Build history of the part. All positions in model axes, mm. Face numbers are marked on the shaded views. A direction names the side the tool comes from. Give positions to 0.01 mm unless a question says otherwise; leave off trailing zeros. Write each loop counter-clockwise with the first axis right and the second up, starting at its lowest first coordinate (ties: lowest second). Pieces come first, ordered by that corner, then holes. Notation, with made-up numbers: (14, 24) -> (35, 24) arc R32 cw to (35, 60) -> close; hole circle Ø1 at (-7, 53). An arc over 180 degrees is marked (long way). One line per question, with ' | ' between items. Start each with the question number.
(1) Tool access for the marked faces 4, 5 and 6: list every direction of +Z, -Z, +X, -X, +Y, -Y with a clear straight run to the whole face (end or side of a thin tool).
(2) Pull direction Z, two halves, no side cores. Call the marked faces 1, 2 and 3: released by +Z, released by -Z, zero draft, split by the parting line, or undercut.
(3) Band-saw the part on A-A, the plane y = -2.25. Give the cut face in (x, z).
(4) Drill centre lines: probe 1 along X at (y, z) = (-2.45, 0); probe 2 along X at (y, z) = (-0.5, 5). Where is each one in solid material? Low to high. Write a range as from..to.
(5) Band-saw the part on B-B, the plane y = 2. Count the separate pieces of the cut face and the enclosed holes in it, and give its area (3 significant figures).
(6) Pin check, flat tips, straight feed: P1, Ø2, axis at x = -0.5, y = 9, coming from the -Z side; P2, Ø1.5, axis at y = 1, z = -6, coming from the -X side; P3, Ø10, axis at x = 13, z = -12, coming from the +Y side; P4, Ø21.5, axis at x = 0.5, z = 3, coming from the -Y side. Stop position of each tip, or through.
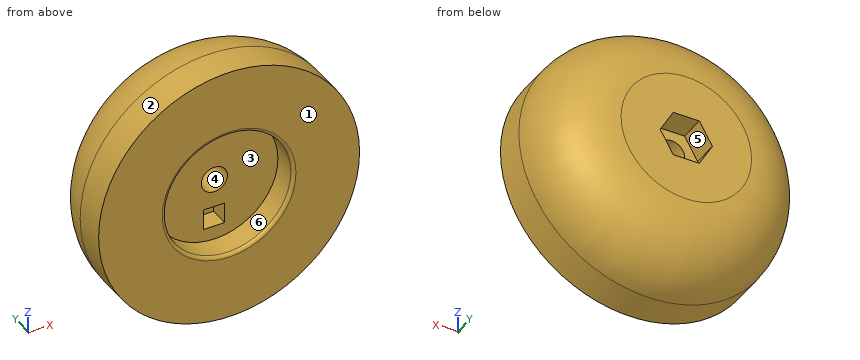
from build123d import *

# Parameters (mm, degrees)
SKETCH1_R           = 9.75
SKETCH1_R_2         = 2
BOSS_EXTRUDE1_DEPTH = 3
SKETCH2_W           = 3.2
SKETCH2_H           = 3.2
CUT_EXTRUDE1_DEPTH  = 3
SKETCH3_R           = 20
BOSS_EXTRUDE2_DEPTH = 8
SKETCH4_R           = 20
SKETCH4_R_2         = 9.75
BOSS_EXTRUDE3_DEPTH = 7
FILLET2_R           = 10
SKETCH5_R           = 2
CUT_EXTRUDE2_DEPTH  = 9
CUT_EXTRUDE3_DEPTH  = 4
FILLET3_R           = 0.5


with BuildPart() as part:
    # Sketch1 → Boss-Extrude1 (new body)
    with BuildSketch(Plane(origin=(0, 0, 0), x_dir=(1, 0, 0), z_dir=(0, 1, 0))):
        Circle(SKETCH1_R)
        Circle(SKETCH1_R_2, mode=Mode.SUBTRACT)
    extrude(amount=BOSS_EXTRUDE1_DEPTH)

    # Sketch2 → Cut-Extrude1 (cut)
    with BuildSketch(Plane.XZ):
        with Locations((-0.030329448, -6.016441714)):
            Rectangle(SKETCH2_W, SKETCH2_H)
    extrude(amount=-CUT_EXTRUDE1_DEPTH, mode=Mode.SUBTRACT)

    # Sketch3 → Boss-Extrude2 (add)
    with BuildSketch(Plane(origin=(0, 3, 0), x_dir=(1, 0, 0), z_dir=(0, 1, 0))):
        Circle(SKETCH3_R)
    extrude(amount=BOSS_EXTRUDE2_DEPTH)

    # Sketch4 → Boss-Extrude3 (add)
    with BuildSketch(Plane.XZ.offset(-3)):
        Circle(SKETCH4_R)
        Circle(SKETCH4_R_2, mode=Mode.SUBTRACT)
    extrude(amount=BOSS_EXTRUDE3_DEPTH)

    # Fillet2
    fillet2_edges = [part.edges().sort_by_distance(p)[0] for p in [
        (-20, 11, 0),
    ]]
    fillet(fillet2_edges, radius=FILLET2_R)

    # Sketch5 → Cut-Extrude2 (cut, through all)
    with BuildSketch(Plane.XZ.offset(-3)):
        Circle(SKETCH5_R)
    extrude(amount=-CUT_EXTRUDE2_DEPTH, mode=Mode.SUBTRACT)

    # Sketch6 → Cut-Extrude3 (cut)
    with BuildSketch(Plane(origin=(0, 11, 0), x_dir=(1, 0, 0), z_dir=(0, 1, 0))):
        Polygon((4.001037365, 0), (2.000518683, 3.465), (-2.000518683, 3.465), (-4.001037365, 0), (-2.000518683, -3.465), (2.000518683, -3.465), align=None)
    extrude(amount=-CUT_EXTRUDE3_DEPTH, mode=Mode.SUBTRACT)

    # Fillet3
    fillet3_edges = [part.edges().sort_by_distance(p)[0] for p in [
        (-9.75, -4, 0),
    ]]
    fillet(fillet3_edges, radius=FILLET3_R)


solid = part.part
Results:
1) face 4: +Y, -Y | face 5: +Y | face 6: -Y
2) face 1: zero draft | face 2: split by the parting line | face 3: undercut
3) outline: circle Ø40 at (0, 0); hole circle Ø19.5 at (0, 0)
4) probe 1: x = -20..-9.75, 9.75..20 | probe 2: x = -19.36..-8.37, 8.37..19.36
5) separate pieces: 1 | enclosed holes: 2 | area: 1,230 mm²
6) P1: stops at z = -17.13 | P2: stops at x = -19.3 | P3: stops at y = 10.63 | P4: stops at y = -4
